Geometry check sheet. Reference: the model listing, model coordinates, mm. A direction names the side the tool comes from. Give positions to 0.01 mm unless a question says otherwise; leave off trailing zeros. Write each loop counter-clockwise with the first axis right and the second up, starting at its lowest first coordinate (ties: lowest second). Pieces come first, ordered by that corner, then holes. Notation, with made-up numbers: (45.25, 26) -> (94.25, 26) arc R19 cw to (94.25, 32) -> close; hole circle Ø6 at (1, 58). An arc over 180 degrees is marked (long way). Write item = value, one per line. Start each with the question number.
1. Thickness scan on line 1 along Y through (x, z) = (-19, 4); line 2 along Y through (x, z) = (-0.25, 2); line 3 along Z through (x, y) = (-14.25, -12.6). Record the ranges inside material, lowest first.
2. Mould release check, pull along Z, two halves, no side actions. Record for faces 1 (the flat face through (-11.5, -11.5, 6.2)), 2 (the cylindrical face through (-20.5, -12.2, 6.4)), 3 (the cylindrical face through (-12.104, -12.26, 6.926)): pulls with the +Z half, pulls with the -Z half, needs draft (parallel to the pull), parting line crosses it, or undercut.
3. Cross-section at B-B, the plane z = 2.5. Record the cut outline in (x, y), plus the area to 4 significant figures.
4. Cross-section at D-D, the plane x = -15. Record the cut outline in (y, z), plus the area to 3 significant figures.
5. Cross-section at C-C, the plane y = 0. Record the cut outline in (x, z), plus the area to 3 significant figures.
6. Depth check by flat-ended pin: P1, Ø5, axis at y = 9, z = 10.5, coming from the +X side; P2, Ø8, axis at x = 2, y = -1.5, coming from the +Z side; P3, Ø0.8, axis at y = 3, z = 1, coming from the -X side. Enter the tip coordinate at first touch or a pass-through.
7. Cross-section at A-A, the plane x = -10. Record the cut outline in (y, z).
8. Set-up check for faces 4 (the flat face through (-11.5, 11.5, 6.2)), 5 (the flat face through (2, -10, 5)), 6 (the flat face through (1.47, -11.48, 8.62)), 7 (the flat face through (-8, 0, 1)): record each of +Z, -Z, +X, -X, +Y, -Y from which the full face is reachable in a straight line by a thin tool's end or side.
```python
from build123d import *

# Parameters (mm, degrees)
SKETCH1_W                    = 16
SKETCH1_H                    = 20
BOSS_EXTRUDE1_DEPTH          = 1.5
BOSS_EXTRUDE2_DEPTH          = 3
CUT_EXTRUDE1_DEPTH           = 1.5
F_4_5_4_5_DIAMETER_HOLE1_D   = 4.5
F_3_0_3_DIAMETER_HOLE1_D     = 3
F_3_0_3_DIAMETER_HOLE1_DEPTH = 12.5


with BuildPart() as part:
    # Sketch1 → Boss-Extrude1 (new body)
    with BuildSketch(Plane(origin=(0, 0, 0), x_dir=(-1, 0, 0), z_dir=(0, 0, -1))):
        Rectangle(SKETCH1_W, SKETCH1_H)
    extrude(amount=-BOSS_EXTRUDE1_DEPTH)

    # Sketch2 → Boss-Extrude2 (add)
    with BuildSketch(Plane(origin=(0, 10, 0), x_dir=(-1, 0, 0), z_dir=(0, 1, 0))):
        with BuildLine():
            Line((14.25, 0), (-8, 0))
            Line((-8, 0), (-8, 4.850108933))
            Line((-8, 4.850108933), (5.25, 12.5))
            Line((5.25, 12.5), (14.25, 12.5))
            ThreePointArc((14.25, 12.5), (20.5, 6.25), (14.25, 0))
        make_face()
    boss_extrude2 = extrude(amount=BOSS_EXTRUDE2_DEPTH)

    # Mirror1: Boss-Extrude2 across plane
    add(boss_extrude2.mirror(Plane.ZX))

    # Sketch4 → Cut-Extrude1 (cut)
    with BuildSketch(Plane(origin=(0, 10, 0), x_dir=(1, 0, 0), z_dir=(0, 1, 0))):
        Polygon((-20.5, -12.5), (-2.25, -12.5), (-2.25, -1.5), (-8, -1.5), (-8, 0), (-20.5, 0), align=None)
    cut_extrude1 = extrude(amount=CUT_EXTRUDE1_DEPTH, mode=Mode.SUBTRACT)

    # Mirror2: Cut-Extrude1 across plane
    add(cut_extrude1.mirror(Plane.ZX), mode=Mode.SUBTRACT)

    # Ø4.5 (4.5) Diameter Hole1 (through all)
    with Locations(Plane(origin=(0, 13, 0), x_dir=(-1, 0, 0), z_dir=(0, 1, 0))):
        with Locations((14.25, 6.25)):
            f_4_5_4_5_diameter_hole1 = Hole(F_4_5_4_5_DIAMETER_HOLE1_D / 2)

    # Mirror3: Ø4.5 (4.5) Diameter Hole1 across plane
    add(f_4_5_4_5_diameter_hole1.mirror(Plane.ZX), mode=Mode.SUBTRACT)

    # Ø3.0 (3) Diameter Hole1
    with Locations(Plane(origin=(0, 0, 0), x_dir=(-1, 0, 0), z_dir=(0, 0, -1))):
        with Locations((-4, 0), (4, 0)):
            Hole(F_3_0_3_DIAMETER_HOLE1_D / 2, depth=F_3_0_3_DIAMETER_HOLE1_DEPTH)


solid = part.part
```
Answers:
q1.line_1 = -13 to -11.5, 11.5 to 13
q1.line_2 = -13 to -10, 10 to 13
q1.line_3 = 0 to 4, 8.5 to 12.5
q2.face_1 = needs draft
q2.face_2 = parting line crosses it
q2.face_3 = undercut
q3.outline = (-19.25, -13) -> (8, -13) -> (8, -10) -> (-2.25, -10) -> (-2.25, -11.5) -> (-19.25, -11.5) -> close; (-19.25, 11.5) -> (-2.25, 11.5) -> (-2.25, 10) -> (8, 10) -> (8, 13) -> (-19.25, 13) -> close
q3.area = 112.5 mm^2
q4.outline = (-13, 0.05) -> (-11.5, 0.05) -> (-11.5, 4.13) -> (-13, 4.13) -> close; (-13, 8.37) -> (-11.5, 8.37) -> (-11.5, 12.45) -> (-13, 12.45) -> close; (11.5, 0.05) -> (13, 0.05) -> (13, 4.13) -> (11.5, 4.13) -> close; (11.5, 8.37) -> (13, 8.37) -> (13, 12.45) -> (11.5, 12.45) -> close
q4.area = 24.5 mm^2
q5.outline = (-8, 0) -> (-5.5, 0) -> (-5.5, 1.5) -> (-8, 1.5) -> close; (-2.5, 0) -> (2.5, 0) -> (2.5, 1.5) -> (-2.5, 1.5) -> close; (5.5, 0) -> (8, 0) -> (8, 1.5) -> (5.5, 1.5) -> close
q5.area = 15.0 mm^2
q6.P1 = 2.18
q6.P2 = 1.5
q6.P3 = -8
q7.outline = (-13, 0) -> (-11.5, 0) -> (-11.5, 12.5) -> (-13, 12.5) -> close; (11.5, 0) -> (13, 0) -> (13, 12.5) -> (11.5, 12.5) -> close
q8.face_4 = +Z, -X
q8.face_5 = +Z, +X, -X
q8.face_6 = +Z, +X, +Y, -Y
q8.face_7 = +Z, -Z, -X
